```python
from build123d import *

# Parameters (mm, degrees)
SKETCH_1_W            = 32
SKETCH_1_H            = 69.6
EXTRUDE_1_DEPTH       = 23
SKETCH_2_R            = 1.5
EXTRUDE_2_DEPTH       = 35
SKETCH_3_W            = 2
SKETCH_3_H            = 3.6
EXTRUDE_3_DEPTH       = 4.5
SKETCH_5_W            = 16
SKETCH_5_H            = 23
CUT_EXTRUDE_1_DEPTH   = 71.5
SKETCH_6_W            = 4.5
SKETCH_6_H            = 3.6
CUT_EXTRUDE_2_DEPTH   = 1
SKETCH_7_W            = 2
SKETCH_7_H            = 4.4
EXTRUDE_4_DEPTH       = 6.5
SKETCH_9_W            = 1
SKETCH_9_H            = 1.8
CUT_EXTRUDE_3_DEPTH   = 4.5
MIRROR_4_OUTLINE_W    = 4.5
MIRROR_4_OUTLINE_H    = 1.8
MIRROR_4_DEPTH        = 1
MIRROR_4_2_OUTLINE_W  = 6.5
MIRROR_4_2_OUTLINE_H  = 4.4
MIRROR_4_2_DEPTH      = 2
SKETCH_10_W           = 1.5
SKETCH_10_H           = 2
EXTRUDE_5_DEPTH       = 4.5
MIRROR_START          = 34.279062003
MIRROR_25_OUTLINE_W   = 69.6
MIRROR_25_OUTLINE_H   = 23
MIRROR_25_DEPTH       = 16
MIRROR_START_2        = -0.720937997
MIRROR_25_2_OUTLINE_R = 1.5
MIRROR_25_2_DEPTH     = 35
MIRROR_START_3        = 27.779062003
MIRROR_25_3_OUTLINE_W = 4.4
MIRROR_25_3_OUTLINE_H = 2
MIRROR_25_3_DEPTH     = 6.5
MIRROR_25_4_OUTLINE_W = 4.5
MIRROR_25_4_OUTLINE_H = 2
MIRROR_25_4_DEPTH     = 1.5
SKETCH_12_W           = 2
SKETCH_12_H           = 4.395113111
EXTRUDE_6_DEPTH       = 7.5
SKETCH_15_W           = 2
SKETCH_15_H           = 3.6
EXTRUDE_7_DEPTH       = 6
SKETCH_14_R           = 1.801767182
CUT_EXTRUDE_4_DEPTH   = 6
SKETCH_17_W           = 2
SKETCH_17_H           = 4.5
EXTRUDE_8_DEPTH       = 6
SKETCH_16_R           = 1.798109405
CUT_EXTRUDE_5_DEPTH   = 6


# Read off the part's stored shape, not the designer's step: ﾐﾗｰ4, ﾐﾗｰ25
with BuildPart() as part:
    # ｽｹｯﾁ1 → ﾎﾞｽ - 押し出し1 (new body)
    with BuildSketch(Plane.XY):
        with Locations((50.279062003, -5.527058824)):
            Rectangle(SKETCH_1_W, SKETCH_1_H)
    extrude(amount=EXTRUDE_1_DEPTH)

    # ｽｹｯﾁ2 → ﾎﾞｽ - 押し出し2 (add)
    with BuildSketch(Plane(origin=(66.279062003, 0, 0), x_dir=(0, 0, -1), z_dir=(1, 0, 0))):
        with Locations(Location((-11.5, -27.627058824, 0), (0, 0, 180))):
            Circle(SKETCH_2_R)
    extrude(amount=EXTRUDE_2_DEPTH)

    # ｽｹｯﾁ3 → ﾎﾞｽ - 押し出し3 (add)
    with BuildSketch(Plane(origin=(66.279062003, 0, 0), x_dir=(0, 0, -1), z_dir=(1, 0, 0))):
        with Locations((-1, -21.322089651)):
            Rectangle(SKETCH_3_W, SKETCH_3_H)
    extrude(amount=EXTRUDE_3_DEPTH)

    # ｽｹｯﾁ5 → ｶｯﾄ - 押し出し1 (cut)
    with BuildSketch(Plane(origin=(0, 29.272941176, 0), x_dir=(1, 0, 0), z_dir=(0, 1, 0))):
        with Locations((42.279062003, -11.5)):
            Rectangle(SKETCH_5_W, SKETCH_5_H)
    extrude(amount=-CUT_EXTRUDE_1_DEPTH, mode=Mode.SUBTRACT)

    # ｽｹｯﾁ6 → ｶｯﾄ - 押し出し2 (cut)
    with BuildSketch(Plane.XY.offset(2)):
        with Locations((68.529062003, -21.322089651)):
            Rectangle(SKETCH_6_W, SKETCH_6_H)
    extrude(amount=-CUT_EXTRUDE_2_DEPTH, mode=Mode.SUBTRACT)

    # ｽｹｯﾁ7 → ﾎﾞｽ - 押し出し4 (add)
    with BuildSketch(Plane(origin=(66.279062003, 0, 0), x_dir=(0, 0, -1), z_dir=(1, 0, 0))):
        with Locations((-1, -17.322089651)):
            Rectangle(SKETCH_7_W, SKETCH_7_H)
    extrude(amount=EXTRUDE_4_DEPTH)

    # ｽｹｯﾁ9 → ｶｯﾄ - 押し出し3 (cut)
    with BuildSketch(Plane(origin=(70.779062003, 0, 0), x_dir=(0, 0, -1), z_dir=(1, 0, 0))):
        with Locations((-0.5, -22.222089651)):
            Rectangle(SKETCH_9_W, SKETCH_9_H)
    extrude(amount=-CUT_EXTRUDE_3_DEPTH, mode=Mode.SUBTRACT)

    # ﾐﾗｰ4 outline → ﾐﾗｰ4 (cut)
    with BuildSketch(Plane.XY):
        with Locations((68.529062003, -20.422089651)):
            Rectangle(MIRROR_4_OUTLINE_W, MIRROR_4_OUTLINE_H)
    extrude(amount=MIRROR_4_DEPTH, mode=Mode.SUBTRACT)

    # Mirror 4 2 outline → Mirror 4 2 (add)
    with BuildSketch(Plane.XY):
        with Locations((69.529062003, -25.322089651)):
            Rectangle(MIRROR_4_2_OUTLINE_W, MIRROR_4_2_OUTLINE_H)
    extrude(amount=MIRROR_4_2_DEPTH)

    # ｽｹｯﾁ10 → ﾎﾞｽ - 押し出し5 (add)
    with BuildSketch(Plane.XZ.offset(19.522089651)):
        with Locations((72.029062003, 1)):
            Rectangle(SKETCH_10_W, SKETCH_10_H)
    extrude(amount=EXTRUDE_5_DEPTH)

    # ﾐﾗｰ25 outline → ﾐﾗｰ25 (add)
    with BuildSketch(Plane.YZ.offset(MIRROR_START)):
        with Locations((-5.527058824, 11.5)):
            Rectangle(MIRROR_25_OUTLINE_W, MIRROR_25_OUTLINE_H)
    extrude(amount=MIRROR_25_DEPTH)

    # Mirror 25 2 outline → Mirror 25 2 (add)
    with BuildSketch(Plane.YZ.offset(MIRROR_START_2)):
        with Locations((-27.627058824, 11.5)):
            Circle(MIRROR_25_2_OUTLINE_R)
    extrude(amount=MIRROR_25_2_DEPTH)

    # Mirror 25 3 outline → Mirror 25 3 (add)
    with BuildSketch(Plane.YZ.offset(MIRROR_START_3)):
        with Locations((-17.322089651, 1)):
            Rectangle(MIRROR_25_3_OUTLINE_W, MIRROR_25_3_OUTLINE_H)
    extrude(amount=MIRROR_25_3_DEPTH)

    # Mirror 25 4 outline → Mirror 25 4 (add)
    with BuildSketch(Plane.YZ.offset(MIRROR_START_3)):
        with Locations((-21.772089651, 1)):
            Rectangle(MIRROR_25_4_OUTLINE_W, MIRROR_25_4_OUTLINE_H)
    extrude(amount=MIRROR_25_4_DEPTH)

    # ｽｹｯﾁ12 → ﾎﾞｽ - 押し出し6 (add)
    with BuildSketch(Plane.ZY.offset(-27.779062003)):
        with Locations((1, -26.219646207)):
            Rectangle(SKETCH_12_W, SKETCH_12_H)
    extrude(amount=-EXTRUDE_6_DEPTH)

    # ｽｹｯﾁ15 → ﾎﾞｽ - 押し出し7 (add)
    with BuildSketch(Plane(origin=(66.279062003, 0, 0), x_dir=(0, 0, -1), z_dir=(1, 0, 0))):
        with Locations((-1, -21.322089651)):
            Rectangle(SKETCH_15_W, SKETCH_15_H)
    extrude(amount=EXTRUDE_7_DEPTH)

    # ｽｹｯﾁ14 → ｶｯﾄ - 押し出し4 (cut)
    with BuildSketch(Plane.XY.offset(2)):
        with Locations((69.477294821, -21.322089651)):
            Circle(SKETCH_14_R)
    extrude(amount=-CUT_EXTRUDE_4_DEPTH, mode=Mode.SUBTRACT)

    # ｽｹｯﾁ17 → ﾎﾞｽ - 押し出し8 (add)
    with BuildSketch(Plane.ZY.offset(-34.279062003)):
        with Locations((1, -21.772089651)):
            Rectangle(SKETCH_17_W, SKETCH_17_H)
    extrude(amount=EXTRUDE_8_DEPTH)

    # ｽｹｯﾁ16 → ｶｯﾄ - 押し出し5 (cut)
    with BuildSketch(Plane.XY.offset(2)):
        with Locations((31.077171408, -21.772089651)):
            Circle(SKETCH_16_R)
    extrude(amount=-CUT_EXTRUDE_5_DEPTH, mode=Mode.SUBTRACT)


solid = part.part
```
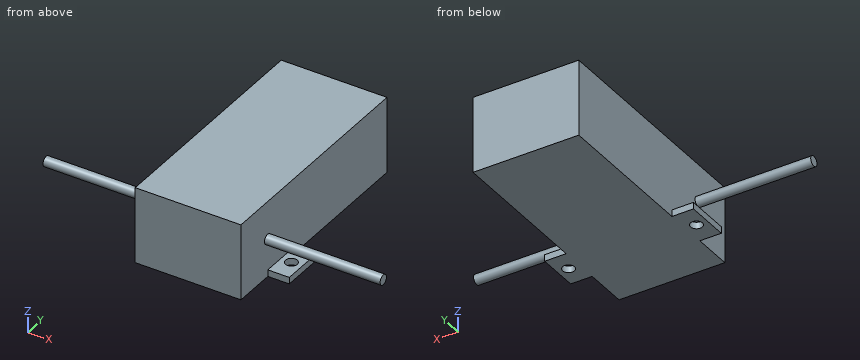
Here's how the part is built. I have some questions about the finished solid (model axes, mm). Give positions to 0.01 mm unless a question says otherwise; leave off trailing zeros. Loops run counter-clockwise (first coordinate to the right, second up) from the corner with the lowest first, then second, coordinate; pieces in that order, holes last. Notation, with made-up numbers: (-16, 52) -> (-5, 52) arc R13 ccw to (-5, 58) -> close; hole circle Ø5 at (-39.5, -10.5). An arc over 180 degrees is marked (long way). Use one line per item in the form item = value. Start each with the question number.
1) For P1, Ø11.5, axis at y = 4.5, z = 12, coming from the -X side; P2, Ø3, axis at y = -9.5, z = 14.5, coming from the +X side; P3, Ø2, axis at x = 69, z = 1, coming from the +Y side; P4, Ø3, axis at x = 69.48, y = -21.32, coming from the -Z side, each with a flat end and sliding along its axis, tell me the tip position at first contact or that it passes through.
2) Please list where these lines run through material, in increasing order: line 1 along X through (y, z) = (-13, 2.75); line 2 along Y through (x, z) = (16, 10.25).
3) Imagine slicing it at A-A (z = 11.5). Please give me the cut outline in (x, y).
4) Imagine slicing it at D-D (z = 16.5). Please give me the cut outline in (x, y).
5) Imagine slicing it at B-B (y = -31). Please give me the cut outline in (x, z), then the cut area to 3 significant figures.
6) Imagine slicing it at C-C (x = 81.5). Please give me the cut outline in (y, z), then the cut area to 3 significant figures.
Check values:
q1.P1 = 34.28
q1.P2 = 66.28
q1.P3 = -15.12
q1.P4 = through
q2.line_1 = 34.28 to 66.28
q2.line_2 = -28.46 to -26.8
q3.outline = (-0.72, -29.13) -> (34.28, -29.13) -> (34.28, -40.33) -> (66.28, -40.33) -> (66.28, -29.13) -> (101.28, -29.13) -> (101.28, -26.13) -> (66.28, -26.13) -> (66.28, 29.27) -> (34.28, 29.27) -> (34.28, -26.13) -> (-0.72, -26.13) -> close
q4.outline = (34.28, -40.33) -> (66.28, -40.33) -> (66.28, 29.27) -> (34.28, 29.27) -> close
q5.outline = (34.28, 0) -> (66.28, 0) -> (66.28, 23) -> (34.28, 23) -> close
q5.area = 736 mm^2
q6.outline = circle Ø3 at (-27.63, 11.5)
q6.area = 7.07 mm^2
